```python
from build123d import *

# Parameters (mm, degrees)
SKETCH1_R           = 1.7
BOSS_EXTRUDE1_DEPTH = 19.05


with BuildPart() as part:
    # Sketch1 → Boss-Extrude1 (new body)
    with BuildSketch(Plane(origin=(0, 0, 0), x_dir=(-1, 0, 0), z_dir=(0, 0, -1))):
        with BuildLine():
            Line((149.085368151, 235.688334746), (149.085368151, 242.188334746))
            ThreePointArc((149.085368151, 242.188334746), (127.872164715, 233.401538181), (119.085368151, 212.188334746))
            Line((119.085368151, 212.188334746), (119.085368151, 96.699570281))
            Line((119.085368151, 96.699570281), (125.585368151, 96.699570281))
            Line((125.585368151, 96.699570281), (125.585368151, 212.188334746))
            ThreePointArc((125.585368151, 212.188334746), (132.468358793, 228.805344103), (149.085368151, 235.688334746))
        make_face()
        with Locations((145.785368151, 238.734002942)):
            Circle(SKETCH1_R, mode=Mode.SUBTRACT)
        with Locations((122.335368151, 212.188334746)):
            Circle(SKETCH1_R, mode=Mode.SUBTRACT)
        with Locations((122.335368151, 156.699570281)):
            Circle(SKETCH1_R, mode=Mode.SUBTRACT)
        with Locations((122.335368151, 100.099570281)):
            Circle(SKETCH1_R, mode=Mode.SUBTRACT)
    extrude(amount=-BOSS_EXTRUDE1_DEPTH)


solid = part.part
```
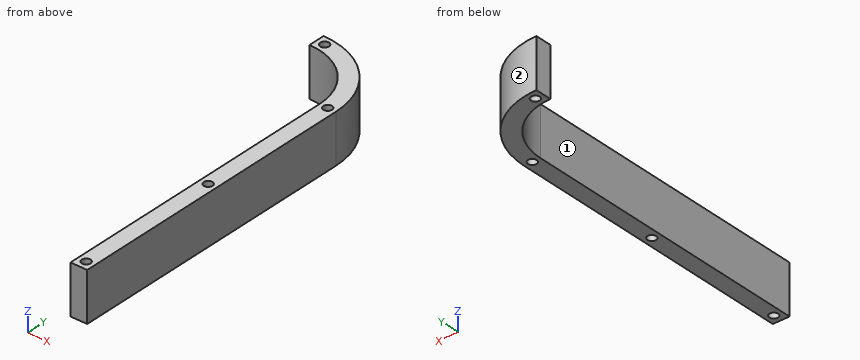
For this review, take the finished solid that the model builds, in its own axes (mm). Face numbers are marked on the shaded views. A direction names the side the tool comes from. Coordinates: 2 decimals unless noted, no trailing zeros. Loops run counter-clockwise (first coordinate to the right, second up) from the corner with the lowest first, then second, coordinate; pieces in that order, holes last.
1. For line 1 (Y direction, x = -123.5, z = 5); line 2 (Y direction, x = -122, z = 7); line 3 (X direction, y = 160.5, z = 4.75), list the stretches that pass through material, from the lowest coordinate up.
2. Add section B-B, the plane y = 117.5. Give the boundary of the cut face in (x, z), then the cut area to 3 significant figures.
3. Add section A-A, the plane z = 14.5. Give the boundary of the cut face in (x, y).
4. Insertion check: P1, Ø4, axis at x = -133, z = 10.5, coming from the -Y side; P2, Ø1.5, axis at x = -127, z = 14, coming from the +Y side; P3, Ø2, axis at x = -122.34, y = 156.7, coming from the -Z side; P4, Ø2, axis at x = -142.5, z = 5.5, coming from the +Y side. Each pin has a flat end and moves straight along its axis. Give the tip position at first contact, or say it passes through.
5. Add section C-C, the plane x = -134.5. Give the boundary of the cut face in (y, z).
6. For the marked faces 1 and 2, list the 3-axis set-ups (+Z, -Z, +X, -X, +Y, -Y) from which the entire face can be reached by the end or side of a thin tool; tool diameter is ignored.
Result:
1. line 1: y = 96.7 to 98.86, 101.34 to 155.46, 157.94 to 210.95, 213.43 to 227.85
1. line 2: y = 96.7 to 98.43, 101.77 to 155.03, 158.37 to 210.52, 213.85 to 225.09
1. line 3: x = -125.59 to -119.09
2. outline: (-125.59, 0) - (-119.09, 0) - (-119.09, 19.05) - (-125.59, 19.05) - close
2. area: 124 mm2
3. outline: (-149.09, 235.69) arc R23.5 cw to (-125.59, 212.19) - (-125.59, 96.7) - (-119.09, 96.7) - (-119.09, 212.19) arc R30 ccw to (-149.09, 242.19) - close; hole circle Ø3.4 at (-145.79, 238.73); hole circle Ø3.4 at (-122.34, 100.1); hole circle Ø3.4 at (-122.34, 156.7); hole circle Ø3.4 at (-122.34, 212.19)
4. P1: stops at y = 227.19
4. P2: stops at y = 233.28
4. P3: passes through
4. P4: stops at y = 241.66
5. outline: (230.61, 0) - (238.4, 0) - (238.4, 19.05) - (230.61, 19.05) - close
6. face 1: +Z, -Z, -X, -Y
6. face 2: +Z, -Z, +X, +Y
